from build123d import *

# Parameters (mm, degrees)
SKETCH1_R           = 7.0625
SKETCH1_R_2         = 4.5625
BOSS_EXTRUDE1_DEPTH = 3
FILLET1_R           = 2
FILLET2_R           = 1


with BuildPart() as part:
    # Sketch1 → Boss-Extrude1 (new body)
    with BuildSketch(Plane.XY):
        with Locations((115.113664311, 46.337958859)):
            Circle(SKETCH1_R)
        with Locations((115.113664311, 46.337958859)):
            Circle(SKETCH1_R_2, mode=Mode.SUBTRACT)
        with BuildLine():
            ThreePointArc((108.051164311, 46.337958859), (110.119722669, 51.331900502), (115.113664311, 53.400458859))
            Line((115.113664311, 53.400458859), (108.051164311, 53.400458859))
            Line((108.051164311, 53.400458859), (108.051164311, 46.337958859))
        make_face()
        with BuildLine():
            Line((108.051164311, 53.400458859), (115.113664311, 53.400458859))
            ThreePointArc((115.113664311, 53.400458859), (120.107605953, 51.331900502), (122.176164311, 46.337958859))
            ThreePointArc((122.176164311, 46.337958859), (121.589956666, 43.520771685), (119.928647546, 41.171253652))
            Line((119.928647546, 41.171253652), (133.051164311, 53.400458859))
            Line((133.051164311, 53.400458859), (133.051164311, 58.400458859))
            Line((133.051164311, 58.400458859), (108.051164311, 58.400458859))
            Line((108.051164311, 58.400458859), (108.051164311, 53.400458859))
        make_face()
    extrude(amount=BOSS_EXTRUDE1_DEPTH)

    # Fillet1
    fillet1_edges = [part.edges().sort_by_distance(p)[0] for p in [
        (108.051164311, 58.400458859, 1.5),
    ]]
    fillet(fillet1_edges, radius=FILLET1_R)

    # Fillet2
    fillet2_edges = [part.edges().sort_by_distance(p)[0] for p in [
        (133.051164311, 58.400458859, 1.5),
        (133.051164311, 53.400458859, 1.5),
    ]]
    fillet(fillet2_edges, radius=FILLET2_R)


solid = part.part
Geometry: final body of the model. Coordinates: model frame, mm. Coordinates: 2 decimals unless noted, no trailing zeros. Order: outer loops, then holes, each group sorted by start corner. A loop starts at its lowest first (then second) coordinate and runs counter-clockwise, first axis right, second up.
(1) Section query B-B (y = 50.25). Return the cut outline in (x, z).
(2) Material intervals for probe 1 along Y at (x, z) = (112.5, 0.65); probe 2 along X at (y, z) = (46.75, 2.1); probe 3 along X at (y, z) = (45.5, 0.9), sorted ascending.
(3) Draft query along X for faces 1 (the face through (133.051, 56, 1)), 2 (the face through (108.051, 51, 1)), 3 (the face through (117.566, 50.185, 1.479)), 4 (the face through (120, 51, 3)). Return one class per face: pulls with the +X half, pulls with the -X half, needs draft (parallel to the pull), parting line crosses it, or undercut.
(4) Section query C-C (x = 114.25). Return the cut outline in (y, z).
(5) Section query D-D (x = 125.75). Return the cut outline in (y, z), plus the area to 3 significant figures.
(6) First-contact query: pin 1 (1 mm diameter, centred on x = 113.5, z = 2.5, fed in from -Y). Flat tip, straight axial feed; report the tip coordinate or a pass-through.
(7) Section query A-A (z = 1.25). Return the cut outline in (x, y) (1 decimal), plus the area to 3 significant figures.
Solution:
1. outline: (108.05, 0) - (112.77, 0) - (112.77, 3) - (108.05, 3) - close; (117.46, 0) - (129.67, 0) - (129.67, 3) - (117.46, 3) - close
2. probe 1: y = 39.78 to 42.6, 50.08 to 58.4
2. probe 2: x = 108.05 to 110.57, 119.66 to 125.91
2. probe 3: x = 108.1 to 110.63, 119.6 to 124.57
3. face 1: pulls with the +X half
3. face 2: pulls with the -X half
3. face 3: undercut
3. face 4: needs draft
4. outline: (39.33, 0) - (41.86, 0) - (41.86, 3) - (39.33, 3) - close; (50.82, 0) - (58.4, 0) - (58.4, 3) - (50.82, 3) - close
5. outline: (46.6, 0) - (58.4, 0) - (58.4, 3) - (46.6, 3) - close
5. area: 35.4 mm2
6. pin 1: stops at y = 39.36
7. outline: (108.1, 46.3) arc R7.1 ccw to (119.9, 41.2) - (132.7, 53.1) arc R1 ccw to (133.1, 53.8) - (133.1, 57.4) arc R1 ccw to (132.1, 58.4) - (110.1, 58.4) arc R2 ccw to (108.1, 56.4) - close; hole circle Ø9.1 at (115.1, 46.3)
7. area: 293 mm2
